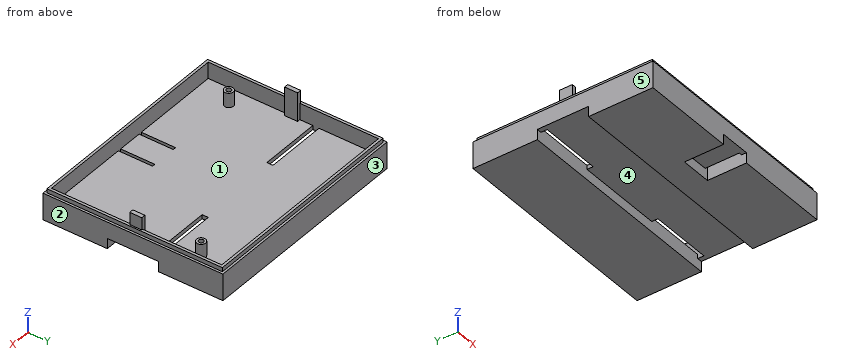
Solid Edge part; units mm, degrees
sketch "Sketch1" plane through (0, 0, 0) normal (0, 0, 1) x (1, 0, 0)
  line L0 (53.5, -43.85) -> (53.5, 43.85)
  line L1 (53.5, 43.85) -> (-53.5, 43.85)
  line L2 (-53.5, 43.85) -> (-53.5, -43.85)
  line L3 (-53.5, -43.85) -> (53.5, -43.85)
extrude "Protrusion1" add sketch "Sketch1" along normal blind 15
sketch "Sketch2" plane through (0, -43.85, 7.5) normal (0, -1, 0) x (1, 0, 0)
  line L0 (7.5, -2.5) -> (-7.5, -2.5)
  line L1 (-7.5, -2.5) -> (-7.5, -12.5)
  line L2 (-7.5, -12.5) -> (7.5, -12.5)
  line L3 (7.5, -12.5) -> (7.5, -2.5)
extrude "VaciadoExtruido_1" cut sketch "Sketch2" against normal blind 19
sketch "Sketch3" plane through (53.5, 0, 7.5) normal (1, 0, 0) x (0, 1, 0)
  line L0 (12.5, -2.5) -> (-12.5, -2.5)
  line L1 (-12.5, -2.5) -> (-12.5, -12.5)
  line L2 (-12.5, -12.5) -> (12.5, -12.5)
  line L3 (12.5, -12.5) -> (12.5, -2.5)
extrude "VaciadoExtruido_2" cut sketch "Sketch3" against normal blind 125.4573
sketch "Sketch4" plane through (0, 0, 15) normal (0, 0, 1) x (1, 0, 0)
  line L0 (51.1, -41.5) -> (51.1, 41.5)
  line L1 (51.1, 41.5) -> (-51.1, 41.5)
  line L2 (-51.1, 41.5) -> (-51.1, -41.5)
  line L3 (-51.1, -41.5) -> (51.1, -41.5)
extrude "VaciadoExtruido_4" cut sketch "Sketch4" against normal blind 8
sketch "Sketch5" plane through (0, 0, 7) normal (0, 0, 1) x (1, 0, 0)
  circle A0 centre (-42.5, -25) radius 2.2
  circle A1 centre (42.5, 25) radius 2.2
extrude "ProtrusiónExtruida_2" add sketch "Sketch5" along normal blind 7
sketch "Sketch6" plane through (0, 0, 7) normal (0, 0, 1) x (-1, 0, 0)
  line L0 (-49.6713, -2.9175) -> (-49.6713, 2.9175)
  line L1 (-49.6713, 2.9175) -> (-51.6713, 2.9175)
  line L2 (-51.6713, 2.9175) -> (-51.6713, -2.9175)
  line L3 (-51.6713, -2.9175) -> (-49.6713, -2.9175)
  line L4 (49.6287, -3.1696) -> (49.6287, 3.1696)
  line L5 (49.6287, 3.1696) -> (51.6287, 3.1696)
  line L6 (51.6287, 3.1696) -> (51.6287, -3.1696)
  line L7 (51.6287, -3.1696) -> (49.6287, -3.1696)
extrude "ProtrusiónExtruida_7" add sketch "Sketch6" along normal blind 14
sketch "Sketch7" plane through (0, 0, 15) normal (0, 0, 1) x (1, 0, 0)
  line L0 (-52.4, 43.85) -> (-52.4, -43.85)
  line L1 (-52.4, -43.85) -> (-53.5, -43.85)
  line L2 (-53.5, -43.85) -> (-53.5, 43.85)
  line L3 (-53.5, 43.85) -> (-52.4, 43.85)
extrude "VaciadoExtruido_12" cut sketch "Sketch7" against normal blind 2
sketch "Sketch8" plane through (0.55, 0, 15) normal (0, 0, 1) x (1, 0, 0)
  line L0 (-52.95, -42.75) -> (52.95, -42.75)
  line L1 (52.95, -42.75) -> (52.95, -43.85)
  line L2 (52.95, -43.85) -> (-52.95, -43.85)
  line L3 (-52.95, -43.85) -> (-52.95, -42.75)
extrude "VaciadoExtruido_14" cut sketch "Sketch8" against normal blind 2
sketch "Sketch9" plane through (0.55, 0.55, 15) normal (0, 0, 1) x (1, 0, 0)
  line L0 (52.95, 43.3) -> (51.85, 43.3)
  line L1 (51.85, 43.3) -> (51.85, -43.3)
  line L2 (51.85, -43.3) -> (52.95, -43.3)
  line L3 (52.95, -43.3) -> (52.95, 43.3)
extrude "VaciadoExtruido_15" cut sketch "Sketch9" against normal blind 2
sketch "Sketch10" plane through (0, 0.55, 15) normal (0, 0, 1) x (1, 0, 0)
  line L0 (-52.4, 43.3) -> (52.4, 43.3)
  line L1 (52.4, 43.3) -> (52.4, 42.2)
  line L2 (52.4, 42.2) -> (-52.4, 42.2)
  line L3 (-52.4, 42.2) -> (-52.4, 43.3)
extrude "VaciadoExtruido_16" cut sketch "Sketch10" against normal blind 2
sketch "Sketch11" plane through (0, 0, 7) normal (0, 0, 1) x (1, 0, 0)
  line L0 (7.5, -41.5) -> (7.5, -24.85)
  line L1 (7.5, -24.85) -> (6, -24.85)
  line L2 (6, -24.85) -> (6, -41.5)
  line L3 (6, -41.5) -> (7.5, -41.5)
  line L4 (-6, -24.85) -> (-6, -41.5)
  line L5 (-6, -41.5) -> (-7.5, -41.5)
  line L6 (-7.5, -41.5) -> (-7.5, -24.85)
  line L7 (-7.5, -24.85) -> (-6, -24.85)
extrude "VaciadoExtruido_17" cut sketch "Sketch11" against normal blind 21
sketch "Sketch12" plane through (0, 0, 7) normal (0, 0, 1) x (1, 0, 0)
  line L0 (-51.1, 12.5) -> (-21.1, 12.5)
  line L1 (-21.1, 12.5) -> (-21.1, 9.5)
  line L2 (-21.1, 9.5) -> (-51.1, 9.5)
  line L3 (-51.1, 9.5) -> (-51.1, 12.5)
  line L4 (51.1, 12.5) -> (21.1, 12.5)
  line L5 (21.1, 12.5) -> (21.1, 9.5)
  line L6 (21.1, 9.5) -> (51.1, 9.5)
  line L7 (51.1, 9.5) -> (51.1, 12.5)
extrude "VaciadoExtruido_18" cut sketch "Sketch12" against normal blind 84
sketch "Sketch13" plane through (-42.5, -25, 14) normal (0, 0, 1) x (1, 0, 0)
  circle A0 centre (0, 0) radius 1.2
  circle A1 centre (85, 50) radius 1.2
extrude "VaciadoExtruido_19" cut sketch "Sketch13" against normal blind 5.5
Source: CAD feature listing. Evaluate the final solid. Frame: model axes, mm. Face numbers are marked on the shaded views. A direction names the side the tool comes from. Coordinates: 2 decimals unless noted, no trailing zeros. Loops run counter-clockwise (first coordinate to the right, second up) from the corner with the lowest first, then second, coordinate; pieces in that order, holes last. Notation, with made-up numbers: (66.5, 55) - (109.5, 55) arc R19 ccw to (109.5, 86) - close; hole circle Ø10 at (27, -28). An arc over 180 degrees is marked (long way). One line per item, written item: value. Start each with the question number.
1. Set-up query: the marked faces 4 and 5. Return all of +Z, -Z, +X, -X, +Y, -Y with unobstructed straight access to the full face (end or side cutting, diameter ignored); none if empty.
2. Ray query, L1, parallel to Y at x = -42.5, z = 11.7; L2, parallel to X at y = -0.5, z = 14.5; L3, parallel to X at y = 21.5, z = 8. Return the intervals inside material, ascending.
3. Section B-B (y = -31). Return the cut outline in (x, z), and give its area (3 significant figures).
4. Mould query, pull axis X, two halves, no side actions, for the marked faces 1, 2 and 3. Classes: pulls with the +X half, pulls with the -X half, needs draft (parallel to the pull), parting line crosses it, or undercut.
5. Section A-A (x = -42.5). Return the cut outline in (y, z).
6. Section C-C (z = 17). Return the cut outline in (x, y).
7. Section D-D (y = -10.5). Return the cut outline in (x, z), and give its area (3 significant figures).
8. Contact query for flat-ended pins moving along their axis: P1, Ø1.6, axis at y = 17.5, z = 14.5, coming from the -X side; P2, Ø3, axis at x = 36.5, y = -19.5, coming from the +Z side; P3, Ø1, axis at x = -17.5, z = 14.5, coming from the -Y side. Output: stop coordinate, or through.
Verdict:
1. face 4: -Z, +X, -X
1. face 5: +Z, -Z, -X, +Y, -Y
2. L1: y = -43.85 to -41.5, -27.2 to -26.2, -23.8 to -22.8, 41.5 to 43.85
2. L2: x = -52.4 to -49.63, 49.67 to 52.4
2. L3: x = -53.5 to -51.1, 51.1 to 53.5
3. outline: (-53.5, 0) - (-7.5, 0) - (-7.5, 7) - (-51.1, 7) - (-51.1, 15) - (-52.4, 15) - (-52.4, 13) - (-53.5, 13) - close; (-6, 5) - (6, 5) - (6, 7) - (-6, 7) - close; (7.5, 0) - (53.5, 0) - (53.5, 13) - (52.4, 13) - (52.4, 15) - (51.1, 15) - (51.1, 7) - (7.5, 7) - close
3. area: 702 mm2
4. face 1: undercut
4. face 2: pulls with the +X half
4. face 3: needs draft
5. outline: (-43.85, 0) - (-12.5, 0) - (-12.5, 5) - (9.5, 5) - (9.5, 7) - (-22.8, 7) - (-22.8, 14) - (-23.8, 14) - (-23.8, 8.5) - (-26.2, 8.5) - (-26.2, 14) - (-27.2, 14) - (-27.2, 7) - (-41.5, 7) - (-41.5, 15) - (-42.75, 15) - (-42.75, 13) - (-43.85, 13) - close; (12.5, 0) - (43.85, 0) - (43.85, 13) - (42.75, 13) - (42.75, 15) - (41.5, 15) - (41.5, 7) - (12.5, 7) - close
6. outline: (-51.63, -3.17) - (-49.63, -3.17) - (-49.63, 3.17) - (-51.63, 3.17) - close; (49.67, -2.92) - (51.67, -2.92) - (51.67, 2.92) - (49.67, 2.92) - close
7. outline: (-53.5, 5) - (53.5, 5) - (53.5, 13) - (52.4, 13) - (52.4, 15) - (51.1, 15) - (51.1, 7) - (-51.1, 7) - (-51.1, 15) - (-52.4, 15) - (-52.4, 13) - (-53.5, 13) - close
7. area: 248 mm2
8. P1: stops at x = -52.4
8. P2: stops at z = 7
8. P3: stops at y = -42.75
